Geometry check sheet. Reference: the model listing, model coordinates, mm. A direction names the side the tool comes from. Give positions to 0.01 mm unless a question says otherwise; leave off trailing zeros. Loops run counter-clockwise (first coordinate to the right, second up) from the corner with the lowest first, then second, coordinate; pieces in that order, holes last.
```python
from build123d import *

# Parameters (mm, degrees)
F0_W     = 82
F0_H     = 126
F1_DEPTH = 35
F2_W     = 80
F2_H     = 124
F3_DEPTH = 5
F4_DEPTH = 1
F5_T     = -1
F6_R     = 2.5
F7_DEPTH = 3


with BuildPart() as f1:
    # F0 (on Top) → F1 (new body)
    with BuildSketch(Plane.XY):
        with Locations((-0.2664038911, -0.5331769297)):
            Rectangle(F0_W, F0_H)
    extrude(amount=F1_DEPTH)

    # F2 (on face) → F3 (cut)
    with BuildSketch(Plane.XY.offset(35)):
        with Locations((-0.2664038911, -0.5331769297)):
            Rectangle(F2_W, F2_H)
    extrude(amount=-F3_DEPTH, mode=Mode.SUBTRACT)

    # F4 (add): a face of the model
    f4_faces = [f1.faces().sort_by_distance(p)[0] for p in [
        (-0.2664038911, -0.5331769297, 30),
    ]]
    extrude(f4_faces, amount=-F4_DEPTH)

    # F5 (hollow: no face is removed)
    offset(amount=F5_T, kind=Kind.INTERSECTION, mode=Mode.SUBTRACT)

    # F6 (on face) → F7 (cut)
    with BuildSketch(Plane(origin=(-41.2664038911, 0, 0), x_dir=(0, -1, 0), z_dir=(-1, 0, 0))):
        with Locations((53.5331769297, 7)):
            Circle(F6_R)
    extrude(amount=-F7_DEPTH, mode=Mode.SUBTRACT)


solid = f1.part
```
1) Sectioned sample at A-A on x = 26. Enter the section's corners in (y, z), plus the area to 3 significant figures.
2) Mould release check, pull along Y, two halves, no side actions. Record for faces 1 (the flat face through (-1, -63.533, 17)), 2 (the flat face through (-1, -62.533, 33)), 3 (the flat face through (-1, 0, 0)): +Y half, -Y half, draft (parallel to the pull), parting line (faces both ways), or undercut.
3) Sectioned sample at B-B on z = 7. Enter the section's corners in (x, y).
4) Scan lines: line 1 along Y through (x, z) = (-2, 19.5); line 2 along Z through (x, y) = (28, -44.5); line 3 along X through (y, z) = (54.5, 9). Record each from-to range of solid material in increasing order.
5) Tool access check on faces 4 (the flat face through (39.734, -1, 33)), 5 (the flat face through (40.734, -1, 17)), 6 (the flat face through (-1, -62.533, 15)), 7 (the cylindrical face through (-40.773, -51.036, 7.11)). Record the directions out of +Z, -Z, +X, -X, +Y, -Y that give a thin tool (end or side, any length) a straight path to the whole face; none if there is none.
6) Sectioned sample at D-D on y = -52.5. Enter the section's corners in (x, z).
7) Sectioned sample at C-C on y = 20.5. Enter the section's corners in (x, z).
8) Depth check by flat-ended pin: P1, Ø12, axis at x = 22.5, y = -30.5, coming from the +Z side; P2, Ø24, axis at x = -16.5, y = 28, coming from the -Z side. Enter the tip coordinate at first touch or a pass-through.
Determined:
1. outline: (-63.53, 0) - (62.47, 0) - (62.47, 35) - (61.47, 35) - (61.47, 30) - (-62.53, 30) - (-62.53, 35) - (-63.53, 35) - close; hole (-62.53, 1) - (61.47, 1) - (61.47, 29) - (-62.53, 29) - close
1. area: 318 mm2
2. face 1: -Y half
2. face 2: undercut
2. face 3: draft
3. outline: (-41.27, -63.53) - (40.73, -63.53) - (40.73, 62.47) - (-41.27, 62.47) - (-41.27, -51.03) - (-40.27, -51.03) - (-40.27, 61.47) - (39.73, 61.47) - (39.73, -62.53) - (-40.27, -62.53) - (-40.27, -56.03) - (-41.27, -56.03) - close
4. line 1: y = -63.53 to -62.53, 61.47 to 62.47
4. line 2: z = 0 to 1, 29 to 30
4. line 3: x = -41.27 to -40.27, 39.73 to 40.73
5. face 4: +Z
5. face 5: +Z, -Z, +X, +Y, -Y
5. face 6: none
5. face 7: -X
6. outline: (-41.27, 0) - (40.73, 0) - (40.73, 35) - (39.73, 35) - (39.73, 30) - (-40.27, 30) - (-40.27, 35) - (-41.27, 35) - (-41.27, 9.28) - (-40.27, 9.28) - (-40.27, 29) - (39.73, 29) - (39.73, 1) - (-40.27, 1) - (-40.27, 4.72) - (-41.27, 4.72) - close
7. outline: (-41.27, 0) - (40.73, 0) - (40.73, 35) - (39.73, 35) - (39.73, 30) - (-40.27, 30) - (-40.27, 35) - (-41.27, 35) - close; hole (-40.27, 1) - (39.73, 1) - (39.73, 29) - (-40.27, 29) - close
8. P1: stops at z = 30
8. P2: stops at z = 0
